Geometry check sheet. Reference: the model listing, model coordinates, mm. A direction names the side the tool comes from. Round coordinates to 2 decimals unless told otherwise and drop trailing zeros. Loops run counter-clockwise (first coordinate to the right, second up) from the corner with the lowest first, then second, coordinate; pieces in that order, holes last.
```python
from build123d import *

# Parameters (mm, degrees)
SKETCH2_R                      = 9.5
SKETCH2_R_2                    = 8.3
CUT_EXTRUDE1_REACH             = 267.847
CUT_EXTRUDE1_DIRECTION_2_REACH = 267.847
CUT_EXTRUDE2_REACH             = 267.847
CUT_EXTRUDE2_END_RADIUS        = 9.5
SKETCH4_R                      = 4
CUT_EXTRUDE3_DEPTH             = 266.846527331
CUT_EXTRUDE3_DEPTH_BACK        = 266.846527331


with BuildPart() as part:
    # Sweep1: sweep along a path in Sketch1
    with BuildLine(Plane.XY) as sweep1_path:
        Line((-21.6, 0), (0, 0))
        Line((0, 0), (185.373442264, 0))
        ThreePointArc((185.373442264, 0), (218.798397967, -12.165688958), (236.58344542, -42.970294761))
        Line((236.58344542, -42.970294761), (240.75, -66.6))
        Line((240.75, -66.6), (243.236210428, -80.7))
    # Sketch2 → Sweep1 (sweep)
    with BuildSketch(Plane.ZY.offset(21.6)):
        Circle(SKETCH2_R)
        Circle(SKETCH2_R_2, mode=Mode.SUBTRACT)
    sweep(path=sweep1_path.line)

    # Sketch3 → Cut-Extrude1 (cut, up to next)
    with BuildSketch(Plane.XY, mode=Mode.PRIVATE) as cut_extrude1_sk1:
        with BuildLine():
            Line((244.802222036, -65.97033418), (244.773201539, -65.805750763))
            ThreePointArc((244.773201539, -65.805750763), (243.33389193, -63.54648723), (240.718605781, -62.966692249))
            Line((240.718605781, -62.966692249), (239.536836478, -63.175070062))
            ThreePointArc((239.536836478, -63.175070062), (237.277572945, -64.614379671), (236.697777964, -67.22966582))
            Line((236.697777964, -67.22966582), (236.726798461, -67.394249237))
            ThreePointArc((236.726798461, -67.394249237), (238.16610807, -69.65351277), (240.781394219, -70.233307751))
            Line((240.781394219, -70.233307751), (241.963163522, -70.024929938))
            ThreePointArc((241.963163522, -70.024929938), (244.222427055, -68.585620329), (244.802222036, -65.97033418))
        make_face()
    cut_extrude1_tool1 = extrude(cut_extrude1_sk1.sketch, amount=-CUT_EXTRUDE1_REACH, mode=Mode.PRIVATE) & part.part
    add(cut_extrude1_tool1.solids().sort_by_distance((240.75, -66.6, 0))[0], mode=Mode.SUBTRACT)

    # Sketch3 → Cut-Extrude1 direction 2 (cut, up to next)
    with BuildSketch(Plane.XY, mode=Mode.PRIVATE) as cut_extrude1_direction_2_sk1:
        with BuildLine():
            Line((244.802222036, -65.97033418), (244.773201539, -65.805750763))
            ThreePointArc((244.773201539, -65.805750763), (243.33389193, -63.54648723), (240.718605781, -62.966692249))
            Line((240.718605781, -62.966692249), (239.536836478, -63.175070062))
            ThreePointArc((239.536836478, -63.175070062), (237.277572945, -64.614379671), (236.697777964, -67.22966582))
            Line((236.697777964, -67.22966582), (236.726798461, -67.394249237))
            ThreePointArc((236.726798461, -67.394249237), (238.16610807, -69.65351277), (240.781394219, -70.233307751))
            Line((240.781394219, -70.233307751), (241.963163522, -70.024929938))
            ThreePointArc((241.963163522, -70.024929938), (244.222427055, -68.585620329), (244.802222036, -65.97033418))
        make_face()
    cut_extrude1_direction_2_tool1 = extrude(cut_extrude1_direction_2_sk1.sketch, amount=CUT_EXTRUDE1_DIRECTION_2_REACH, mode=Mode.PRIVATE) & part.part
    add(cut_extrude1_direction_2_tool1.solids().sort_by_distance((240.75, -66.6, 0))[0], mode=Mode.SUBTRACT)

    # Cut-Extrude2: up to this cylinder (the profile starts inside it)
    cut_extrude2_end = Plane(origin=(0, 0, 0), z_dir=(-1, 0, 0)) * Cylinder(CUT_EXTRUDE2_END_RADIUS, 555.694, mode=Mode.PRIVATE)
    # Sketch4 → Cut-Extrude2 (cut, up to the surface)
    with BuildSketch(Plane.XY, mode=Mode.PRIVATE) as cut_extrude2_sk1:
        with Locations(Location((0, 0, 0), (0, 0, 90))):
            Circle(SKETCH4_R)
    cut_extrude2_tool1 = extrude(cut_extrude2_sk1.sketch, amount=CUT_EXTRUDE2_REACH, mode=Mode.PRIVATE) & cut_extrude2_end
    add(cut_extrude2_tool1.solids().sort_by_distance((0, 0, 0))[0], mode=Mode.SUBTRACT)

    # Sketch5 → Cut-Extrude3 (cut, two sides: drawn at the far end of the back side and taken through both)
    with BuildSketch(Plane.XY.offset(-CUT_EXTRUDE3_DEPTH_BACK)):
        Polygon((-21.6, 0), (-21.6, 2.555), (-16.4, 2.555), (-16.4, -2.555), (-21.6, -2.555), align=None)
    extrude(amount=CUT_EXTRUDE3_DEPTH + CUT_EXTRUDE3_DEPTH_BACK, mode=Mode.SUBTRACT)


solid = part.part
```
1) Sectioned sample at A-A, the plane z = 0. Record the cut outline in (x, y), then the cut area to 3 significant figures.
Report:
outline: (-21.6, -9.5) - (185.37, -9.5) arc R42.5 cw to (227.23, -44.62) - (233.88, -82.35) - (235.06, -82.14) - (228.41, -44.41) arc R43.7 ccw to (185.37, -8.3) - (-21.6, -8.3) - close; (-21.6, 8.3) - (185.37, 8.3) arc R60.3 cw to (244.76, -41.53) - (251.41, -79.26) - (252.59, -79.05) - (245.94, -41.32) arc R61.5 ccw to (185.37, 9.5) - (-21.6, 9.5) - close
area: 763 mm2
2) Mould release check, pull along Z, two halves, no side actions. Record for faces 1 (the face through (83.336, 3.639, 8.776)), 2 (the face through (83.336, 8.103, -1.799)), 3 (the face through (-21.6, -8.4, 1.4)): +Z half, -Z half, draft (parallel to the pull), parting line (faces both ways), or undercut.
Report:
face 1: parting line
face 2: undercut
face 3: draft
3) Scan lines: line 1 along Y through (x, z) = (31, 4); line 2 along Y through (x, z) = (88, 0). Record each from-to range of solid material in increasing order.
Report:
line 1: y = -8.62 to -7.27, 7.27 to 8.62
line 2: y = -9.5 to -8.3, 8.3 to 9.5
4) Gauge pin test, flat ends, axial feed: pin 1 (8 mm diameter, centred on x = 185.5, z = 7, fed in from -Y); pin 2 (3 mm diameter, centred on x = 154.5, z = 6, fed in from -Y); pin 3 (0.6 mm diameter, centred on x = -19, z = 8.5, fed in from -Y). Record the tip position at first contact, or that the pin passes through.
Report:
pin 1: stops at y = -9.01
pin 2: stops at y = -8.37
pin 3: stops at y = -4.8
5) Sectioned sample at C-C, the plane x = 0. Record the cut outline in (y, z), then the cut area to 3 significant figures.
Report:
outline: (-4, 7.27) - (-4, 8.62) arc R9.5 ccw (long way) to (4, 8.62) - (4, 7.27) arc R8.3 cw (long way) to start
area: 57.1 mm2
6) Sectioned sample at B-B, the plane x = 167. Record the cut outline in (y, z), then the cut area to 3 significant figures.
Report:
outline: circle Ø19 at (0, 0); hole circle Ø16.6 at (0, 0)
area: 67.1 mm2
7) Access from +Z, -Z, +X, -X, +Y, -Y to the whole of each face (thin tool, end or side, straight path). Record for faces 4 (the face through (-21.6, 9, 0)), 5 (the face through (-3.966, -0.521, 8.618)).
Report:
face 4: +Z, -Z, -X, +Y, -Y
face 5: +Z
